```python
from build123d import *

# Parameters (mm, degrees)
SKETCH1_R           = 46
SKETCH1_R_2         = 45.25
BOSS_EXTRUDE1_DEPTH = 30
SKETCH3_R           = 47
BOSS_EXTRUDE2_DEPTH = 3
SKETCH4_R           = 2
SKETCH4_R_2         = 8
CUT_EXTRUDE1_DEPTH  = 75.209163855
BOSS_EXTRUDE3_START = 27
SKETCH5_R           = 45.25
SKETCH5_R_2         = 44.5
BOSS_EXTRUDE3_DEPTH = 27


with BuildPart() as part:
    # Sketch1 → Boss-Extrude1 (new body)
    with BuildSketch(Plane(origin=(0, 0, 0), x_dir=(1, 0, 0), z_dir=(0, 1, 0))):
        with Locations(Location((0, 0, 0), (0, 0, 270))):
            Circle(SKETCH1_R)
        with Locations(Location((0, 0, 0), (0, 0, 270))):
            Circle(SKETCH1_R_2, mode=Mode.SUBTRACT)
    extrude(amount=BOSS_EXTRUDE1_DEPTH)

    # Sketch3 → Boss-Extrude2 (add)
    with BuildSketch(Plane(origin=(0, 30, 0), x_dir=(1, 0, 0), z_dir=(0, 1, 0))):
        with Locations(Location((0, 0, 0), (0, 0, 270))):
            Circle(SKETCH3_R)
    extrude(amount=BOSS_EXTRUDE2_DEPTH)

    # Sketch4 → Cut-Extrude1 (cut, through all)
    with BuildSketch(Plane(origin=(0, 33, 0), x_dir=(1, 0, 0), z_dir=(0, 1, 0))):
        with Locations(Location((0, 35, 0), (0, 0, 270))):
            Circle(SKETCH4_R)
        with Locations(Location((0, -35, 0), (0, 0, 270))):
            Circle(SKETCH4_R)
        with Locations(Location((0, 0, 0), (0, 0, 270))):
            Circle(SKETCH4_R_2)
    extrude(amount=-CUT_EXTRUDE1_DEPTH, mode=Mode.SUBTRACT)

    # Sketch5 → Boss-Extrude3 (add)
    with BuildSketch(Plane.XZ.offset(-30).offset(BOSS_EXTRUDE3_START)):
        with Locations(Location((0, 0, 0), (0, 0, 270))):
            Circle(SKETCH5_R)
        with Locations(Location((0, 0, 0), (0, 0, 270))):
            Circle(SKETCH5_R_2, mode=Mode.SUBTRACT)
    extrude(amount=-BOSS_EXTRUDE3_DEPTH)


solid = part.part
```
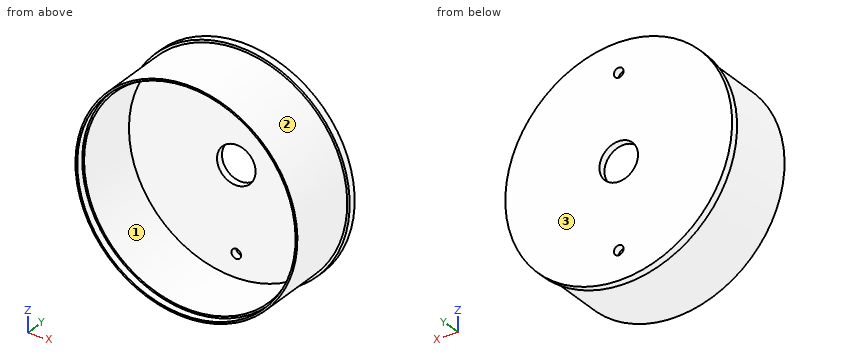
Check sheet for the modelled part. Datum: model origin and axes. Units: mm. Face numbers are marked on the shaded views. Round coordinates to 2 decimals unless told otherwise and drop trailing zeros. Order: outer loops, then holes, each group sorted by start corner. A loop starts at its lowest first (then second) coordinate and runs counter-clockwise, first axis right, second up. Notation, with made-up numbers: M 76,-6 L 128,-6 A27 cw 128,15 Z; hole C 15.5,79.5 d3. An arc over 180 degrees is marked long. Answer in a Markdown table with one row per item.
(1) Gauge pin test, flat ends, axial feed: pin 1 (4 mm diameter, centred on x = -31, y = 11.5, fed in from -Z); pin 2 (6 mm diameter, centred on y = 13.5, z = 17, fed in from -X); pin 3 (9.5 mm diameter, centred on x = 0, z = 0, fed in from -Y); pin 4 (3 mm diameter, centred on x = 27, z = -8.5, fed in from -Y). Record the tip position at first contact, or that the pin passes through.
Findings:
| item | result |
|---|---|
| pin 1 | stops at z = -35.71 |
| pin 2 | stops at x = -43.82 |
| pin 3 | passes through |
| pin 4 | stops at y = 30 |
(2) Section check C-C on y = 7.5. Record the boundary of the cut face in (x, z).
Findings:
| item | result |
|---|---|
| outline | C 0,0 d92; hole C 0,0 d89 |
(3) Material ranges on line 1 along X through (y, z) = (17, 0); line 2 along X through (y, z) = (1.15, 0); line 3 along Y through (x, z) = (20.5, 15.5), recorded low to high. Write a range as from..to.
Findings:
| item | result |
|---|---|
| line 1 | x = -46..-44.5, 44.5..46 |
| line 2 | x = -46..-45.25, 45.25..46 |
| line 3 | y = 30..33 |
(4) Section check D-D on x = -40. Record the boundary of the cut face in (y, z), plus the area to 3 significant figures.
Findings:
| item | result |
|---|---|
| outline | M 0,-22.72 L 30,-22.72 L 30,-24.68 L 33,-24.68 L 33,24.68 L 30,24.68 L 30,22.72 L 0,22.72 L 0,21.16 L 3,21.16 L 3,19.5 L 30,19.5 L 30,-19.5 L 3,-19.5 L 3,-21.16 L 0,-21.16 Z |
| area | 331 mm^2 |
(5) Section check A-A on x = 0. Record the boundary of the cut face in (y, z), plus the area to 4 significant figures.
Findings:
| item | result |
|---|---|
| outline | M 0,-46 L 30,-46 L 30,-47 L 33,-47 L 33,-37 L 30,-37 L 30,-44.5 L 3,-44.5 L 3,-45.25 L 0,-45.25 Z; M 0,45.25 L 3,45.25 L 3,44.5 L 30,44.5 L 30,37 L 33,37 L 33,47 L 30,47 L 30,46 L 0,46 Z; M 30,-33 L 33,-33 L 33,-8 L 30,-8 Z; M 30,8 L 33,8 L 33,33 L 30,33 Z |
| area | 295.5 mm^2 |
(6) Draft check along Z on the marked faces 1, 2 and 3. Enter one of: +Z half, -Z half, draft (parallel to the pull), parting line (faces both ways), or undercut.
Findings:
| item | result |
|---|---|
| face 1 | undercut |
| face 2 | parting line |
| face 3 | draft |
(7) Section check B-B on z = 0. Record the boundary of the cut face in (x, y).
Findings:
| item | result |
|---|---|
| outline | M -47,30 L -46,30 L -46,0 L -45.25,0 L -45.25,3 L -44.5,3 L -44.5,30 L -8,30 L -8,33 L -47,33 Z; M 8,30 L 44.5,30 L 44.5,3 L 45.25,3 L 45.25,0 L 46,0 L 46,30 L 47,30 L 47,33 L 8,33 Z |
